Verification items for this drawing (mm, ordinates from the low corner). A direction names the side the tool comes from. Give positions to 0.01 mm unless a question says otherwise; leave off trailing zeros. Order: outer loops, then holes, each group sorted by start corner. A loop starts at its lowest first (then second) coordinate and runs counter-clockwise, first axis right, second up.
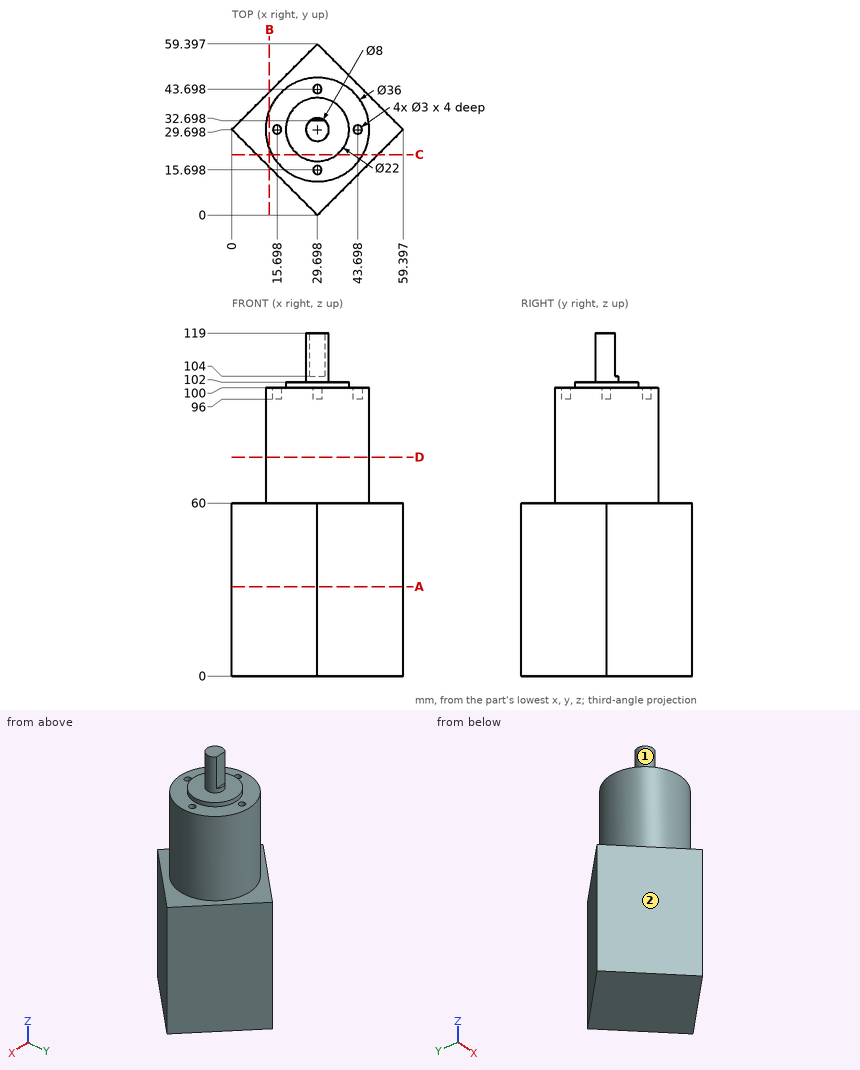
Q1. Gauge pin test, flat ends, axial feed: P1, Ø2, axis at x = 16, z = 57, coming from the -Y side; P2, Ø3.5, axis at x = 43, y = 29.5, coming from the +Z side; P3, Ø5, axis at x = 26.5, y = 19.5, coming from the +Z side. Record the tip position at first contact, or that the pin passes through.
Q2. Cross-section at D-D, the plane z = 76. Record the boundary of the cut face in (x, y).
Q3. Cross-section at B-B, the plane x = 13. Record the boundary of the cut face in (y, z).
Q4. Cross-section at C-C, the plane y = 21. Record the boundary of the cut face in (x, z) (1 decimal).
Q5. Access from +Z, -Z, +X, -X, +Y, -Y to the whole of each face (thin tool, end or side, straight path). Record for the marked faces 1 and 2.
Q6. Cross-section at A-A, the plane z = 31. Record the boundary of the cut face in (x, y).
Q7. Thickness scan on L1, parallel to Z at x = 18.5, y = 28; L2, parallel to Z at x = 33, y = 7; L3, parallel to Y at x = 36.5, z = 53 (1 decimal). Record the ranges inside material, lowest first.
Answers follow:
1. P1: stops at y = 12.7
1. P2: stops at z = 100
1. P3: stops at z = 102
2. outline: circle Ø36 at (29.7, 29.7)
3. outline: (16.7, 0) - (42.7, 0) - (42.7, 60) - (36.42, 60) - (36.42, 100) - (22.98, 100) - (22.98, 60) - (16.7, 60) - close
4. outline: (8.7, 0) - (50.7, 0) - (50.7, 60) - (45.5, 60) - (45.5, 100) - (36.4, 100) - (36.4, 102) - (23, 102) - (23, 100) - (13.9, 100) - (13.9, 60) - (8.7, 60) - close
5. face 1: +Z
5. face 2: +Z, -Z, -X, -Y
6. outline: (0, 29.7) - (29.7, 0) - (59.4, 29.7) - (29.7, 59.4) - close
7. L1: z = 0 to 100
7. L2: z = 0 to 60
7. L3: y = 6.8 to 52.6
